```python
from build123d import *

# Parameters (mm, degrees)
SWEEP2_PROFILE_R = 1.5


with BuildPart() as part:
    # Sweep2: sweep along a path in Sketch1
    with BuildLine(Plane.XY) as sweep2_path:
        Line((27, 0), (32, 0))
        ThreePointArc((32, 0), (33.414213562, 0.585786438), (34, 2))
        Line((34, 2), (34, 22.971251236))
        ThreePointArc((34, 22.971251236), (33.633140648, 24.851146908), (32.586396904, 26.455179657))
        Line((32.586396904, 26.455179657), (3.586396904, 56.308120834))
        ThreePointArc((3.586396904, 56.308120834), (0, 57.824192412), (-3.586396904, 56.308120834))
        Line((-3.586396904, 56.308120834), (-32.586396904, 26.455179657))
        ThreePointArc((-32.586396904, 26.455179657), (-33.633140648, 24.851146908), (-34, 22.971251236))
        Line((-34, 22.971251236), (-34, 2))
        ThreePointArc((-34, 2), (-33.414213562, 0.585786438), (-32, 0))
        Line((-32, 0), (-27, 0))
    # Sweep2 profile (on start of the path) → Sweep2 (sweep)
    with BuildSketch(Plane(origin=(27, 0, 0), x_dir=(0, 0, 1), z_dir=(1, 0, 0))):
        Circle(SWEEP2_PROFILE_R)
    sweep(path=sweep2_path.line)


solid = part.part
```
Work out the finished part from the listing and answer in its coordinate system (mm). A direction names the side the tool comes from. Round coordinates to 2 decimals unless told otherwise and drop trailing zeros. Write each loop counter-clockwise with the first axis right and the second up, starting at its lowest first coordinate (ties: lowest second). Pieces come first, ordered by that corner, then holes.
1) Flat-ended cylindrical pins translate along their axes: P1, Ø1.5, axis at y = 0.5, z = 0.5, coming from the -X side; P2, Ø1, axis at x = 19.5, z = -1, coming from the -Y side; P3, Ø0.9, axis at y = -0.5, z = 0.5, coming from the +X side. Find the tip coordinate at first contact, or state that the pin passes through.
2) Which of the six approach directions +Z, -Z, +X, -X, +Y, -Y give full straight-line access (tool end or side, diameter ignored) to faces 1 (the face through (27, 0, 0)), 2 (the face through (29.54, -0.07, -1.5))?
3) Consider probe 1 along X at (y, z) = (13.5, -0.05); probe 2 along X at (y, z) = (3, 1); probe 3 along Y at (x, z) = (32.5, -0.9). Determine where each line is inside the solid, lowest interval first.
4) A cutting plane is placed at B-B on z = 0. Determine the outline of the cut face in (x, y).
5) A cutting plane is placed at A-A on y = 16.5. Determine the outline of the cut face in (x, z).
Entries:
1. P1: stops at x = -35.39
1. P2: stops at y = 37.61
1. P3: stops at x = 34.77
2. face 1: +Z, -Z, -Y
2. face 2: none
3. probe 1: x = -35.5 to -32.5, 32.5 to 35.5
3. probe 2: x = -35.12 to -32.88, 32.88 to 35.12
3. probe 3: y = -1.16 to 1.38, 24.45 to 28.27
4. outline: (-35.5, 2) arc R3.5 ccw to (-32, -1.5) - (-27, -1.5) - (-27, 1.5) - (-32, 1.5) arc R0.5 cw to (-32.5, 2) - (-32.5, 22.97) arc R3.5 cw to (-31.51, 25.41) - (-2.51, 55.26) arc R3.5 cw to (2.51, 55.26) - (31.51, 25.41) arc R3.5 cw to (32.5, 22.97) - (32.5, 2) arc R0.5 cw to (32, 1.5) - (27, 1.5) - (27, -1.5) - (32, -1.5) arc R3.5 ccw to (35.5, 2) - (35.5, 22.97) arc R6.5 ccw to (33.66, 27.5) - (4.66, 57.35) arc R6.5 ccw to (-4.66, 57.35) - (-33.66, 27.5) arc R6.5 ccw to (-35.5, 22.97) - close
5. outline: circle Ø3 at (-34, 0); circle Ø3 at (34, 0)
